The figure shows three views and two pictorial views of one solid part (mm, origin at its lowest corner). Answer the questions. Round coordinates to 2 decimals unless told otherwise and drop trailing zeros. Loops run counter-clockwise (first coordinate to the right, second up) from the corner with the lowest first, then second, coordinate; pieces in that order, holes last. Notation, with made-up numbers: (35, -2.75) -> (69, -2.75) arc R24 ccw to (69, 35.25) -> close; hole circle Ø4 at (84, 66.5). An arc over 180 degrees is marked (long way). Put each result on its own line as item: value.
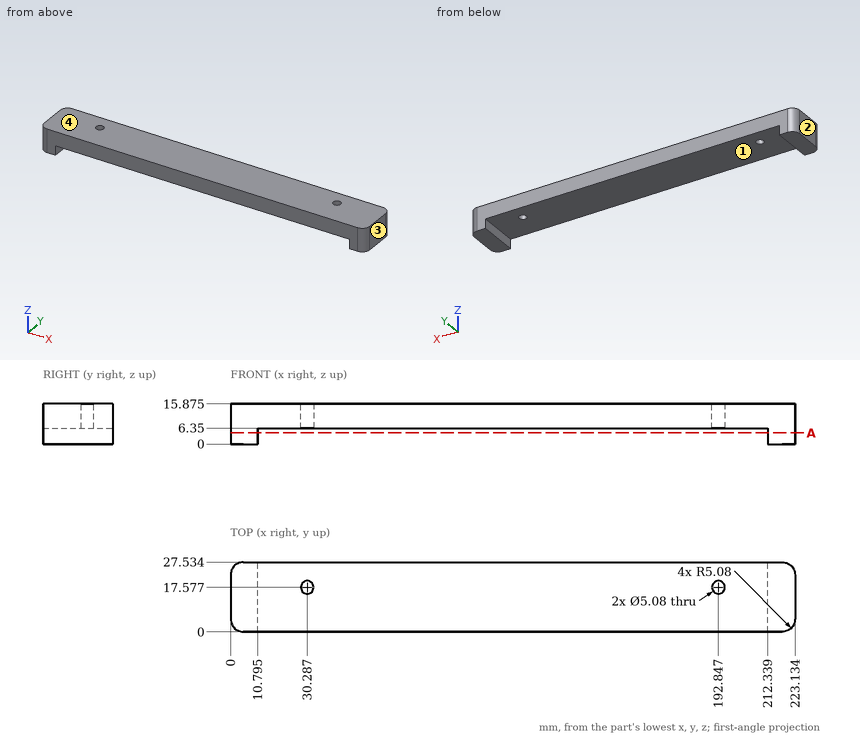
Item 1: Find the intervals of material crossed by line 1 along X through (y, z) = (15.25, 1) (1 decimal); line 2 along X through (y, z) = (18, 12.5); line 3 along X through (y, z) = (19.75, 6.5) (1 decimal), in increasing order.
Derived:
line 1: x = 0 to 10.8, 212.3 to 223.1
line 2: x = 0 to 27.78, 32.79 to 190.34, 195.35 to 223.13
line 3: x = 0 to 29, 31.6 to 191.5, 194.2 to 223.1
Item 2: A flat-ended cylindrical pin translates along its axis: pin 1 Ø12 at (x, y) = (165.5, 18.5) entering from -Z. Find the tip coordinate at first contact, or state that the pin passes through.
Derived:
pin 1: stops at z = 6.35
Item 3: The part is cut by section A-A (z = 4.5). Determine the outline of the cut face in (x, y) (1 decimal).
Derived:
outline: (0, 5.1) arc R5.1 ccw to (5.1, 0) -> (10.8, 0) -> (10.8, 27.5) -> (5.1, 27.5) arc R5.1 ccw to (0, 22.5) -> close; (212.3, 0) -> (218.1, 0) arc R5.1 ccw to (223.1, 5.1) -> (223.1, 22.5) arc R5.1 ccw to (218.1, 27.5) -> (212.3, 27.5) -> close
Item 4: For a pull along X with two mould halves and no side action, classify the marked faces 1, 2, 3 and 4 as pulls with the +X half, pulls with the -X half, needs draft (parallel to the pull), parting line crosses it, or undercut.
Derived:
face 1: undercut
face 2: pulls with the -X half
face 3: pulls with the +X half
face 4: needs draft
